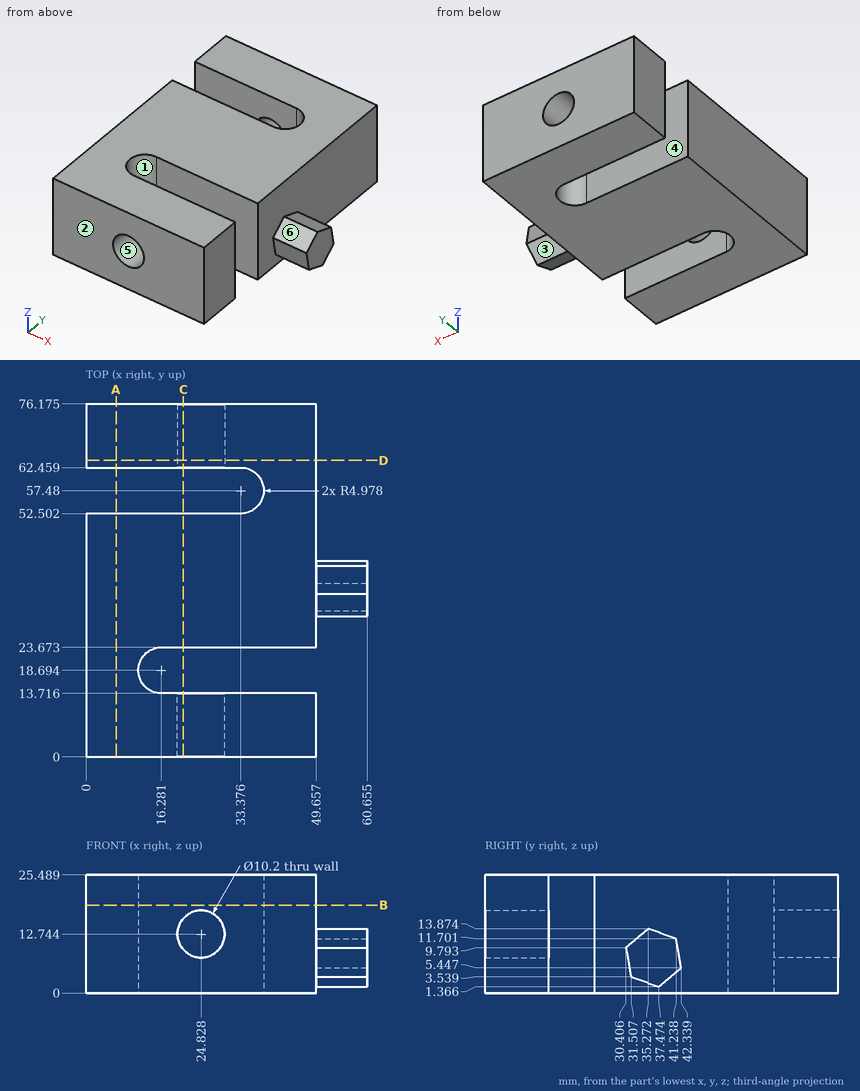
Geometry: see drawing. Coordinates: mm, zero at the bounding-box minimum. A direction names the side the tool comes from. Round coordinates to 2 decimals unless told otherwise and drop trailing zeros. Write each loop counter-clockwise with the first axis right and the second up, starting at its lowest first coordinate (ties: lowest second). Pieces come first, ordered by that corner, then holes. Notation, with made-up numbers: M 11,46.25 L 37,46.25 A15 ccw 37,75.25 Z; hole C -6.75,-1.75 d10. An arc over 180 degrees is marked long. Answer as a JSON object with one key per item and string values. Group by question number.
(1) First-contact query: pin 1 (6 mm diameter, centred on x = 24.83, z = 12.74, fed in from +Y); pin 2 (6 mm diameter, centred on y = 44.5, z = 13, fed in from +X); pin 3 (9 mm diameter, centred on x = 24.83, z = 12.74, fed in from -Y). Flat tips, straight axial feed; report the tip coordinate or a pass-through.
(2) Ray query, line 1 (Y direction, x = 29.5, z = 22.75) (1 decimal); line 2 (Y direction, x = 48.5, z = 14.5) (1 decimal); line 3 (Y direction, x = 6.5, z = 11.75) (1 decimal). Return the intervals inside material, ascending. Write a range as [from, to].
(3) Section query C-C on x = 21. Output: boundary loops of the cut face in (y, z) (1 decimal), then the cut area to 3 significant figures.
(4) Reachability of the marked faces 4, 5 and 6 from +Z, -Z, +X, -X, +Y, -Y: full face, straight path, thin tool, end or side. Return the list, or none.
(5) Mould query, pull axis Y, two halves, no side actions, for the marked faces 1, 2 and 3. Classes: +Y half, -Y half, draft (parallel to the pull), parting line (faces both ways), or undercut.
(6) Section query A-A on x = 6.5. Output: boundary loops of the cut face in (y, z) (1 decimal), then the cut area to 3 significant figures.
(7) Section query D-D on y = 64. Output: boundary loops of the cut face in (x, z) (1 decimal), then the cut area to 3 significant figures.
(8) Section query B-B on z = 19. Output: boundary loops of the cut face in (x, y) (1 decimal), then the cut area to 3 significant figures.
Computed values:
{
 "1": {"pin 1": "y = 52.5", "pin 2": "x = 49.66", "pin 3": "y = 23.67"},
 "2": {"line 1": "[0, 13.7], [23.7, 52.5], [62.5, 76.2]", "line 2": "[0, 13.7], [23.7, 76.2]", "line 3": "[0, 52.5], [62.5, 76.2]"},
 "3": {"outline": "M 0,0 L 13.7,0 L 13.7,9.4 L 0,9.4 Z; M 0,16.1 L 13.7,16.1 L 13.7,25.5 L 0,25.5 Z; M 23.7,0 L 52.5,0 L 52.5,25.5 L 23.7,25.5 Z; M 62.5,0 L 76.2,0 L 76.2,9.4 L 62.5,9.4 Z; M 62.5,16.1 L 76.2,16.1 L 76.2,25.5 L 62.5,25.5 Z", "area": "1,250 mm^2"},
 "4": {"face 4": "+Z, -Z, -X", "face 5": "-Y", "face 6": "+Z, +X, -Y"},
 "5": {"face 1": "undercut", "face 2": "-Y half", "face 3": "+Y half"},
 "6": {"outline": "M 0,0 L 52.5,0 L 52.5,25.5 L 0,25.5 Z; M 62.5,0 L 76.2,0 L 76.2,25.5 L 62.5,25.5 Z", "area": "1,690 mm^2"},
 "7": {"outline": "M 0,0 L 49.7,0 L 49.7,25.5 L 0,25.5 Z; hole C 24.8,12.7 d10.2", "area": "1,180 mm^2"},
 "8": {"outline": "M 0,0 L 49.7,0 L 49.7,13.7 L 16.3,13.7 A5 cw 16.3,23.7 L 49.7,23.7 L 49.7,76.2 L 0,76.2 L 0,62.5 L 33.4,62.5 A5 cw 33.4,52.5 L 0,52.5 Z", "area": "3,040 mm^2"}
}
